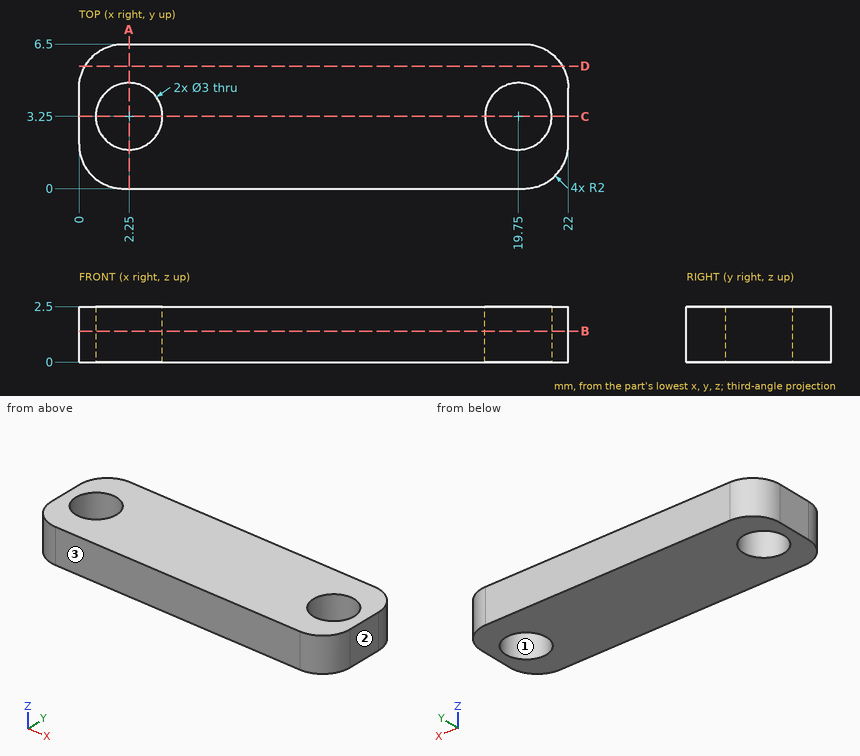
Design review of the part shown in the three views and the two pictorial views. Dimensions are in mm from the part's minimum x, y and z. Give positions to 0.01 mm unless a question says otherwise; leave off trailing zeros. Write each loop counter-clockwise with the first axis right and the second up, starting at its lowest first coordinate (ties: lowest second). Pieces come first, ordered by that corner, then holes. Notation, with made-up numbers: M 65,35.25 L 74,35.25 A26 cw 74,71.25 Z; hole C 1.5,58 d1. An arc over 180 degrees is marked long. Answer in a Markdown table with one row per item.
Item 1: For P1, Ø2.5, axis at x = 19.75, y = 3.25, coming from the -Z side, flat-tipped, find the tip position at first contact; note if it passes through.
Check sheet entries:
| item | result |
|---|---|
| P1 | through |
Item 2: Draft analysis for pull direction Y (two halves, no side actions). For the marked faces 1, 2 and 3, state which applies: +Y half, -Y half, draft (parallel to the pull), parting line (faces both ways), or undercut.
Check sheet entries:
| item | result |
|---|---|
| face 1 | undercut |
| face 2 | draft |
| face 3 | -Y half |
Item 3: Add section B-B on z = 1.4. Give the boundary of the cut face in (x, y).
Check sheet entries:
| item | result |
|---|---|
| outline | M 0,2 A2 ccw 2,0 L 20,0 A2 ccw 22,2 L 22,4.5 A2 ccw 20,6.5 L 2,6.5 A2 ccw 0,4.5 Z; hole C 2.25,3.25 d3; hole C 19.75,3.25 d3 |
Item 4: For line 1 along Y through (x, z) = (19.75, 0.75); line 2 along X through (y, z) = (2.75, 0.75); line 3 along Y through (x, z) = (18.5, 0.65), list the stretches that pass through material, from the lowest coordinate up.
Check sheet entries:
| item | result |
|---|---|
| line 1 | 0 to 1.75, 4.75 to 6.5 |
| line 2 | 0 to 0.84, 3.66 to 18.34, 21.16 to 22 |
| line 3 | 0 to 2.42, 4.08 to 6.5 |
Item 5: Add section C-C on y = 3.25. Give the boundary of the cut face in (x, z), plus the area to 3 significant figures.
Check sheet entries:
| item | result |
|---|---|
| outline | M 0,0 L 0.75,0 L 0.75,2.5 L 0,2.5 Z; M 3.75,0 L 18.25,0 L 18.25,2.5 L 3.75,2.5 Z; M 21.25,0 L 22,0 L 22,2.5 L 21.25,2.5 Z |
| area | 40.0 mm2 |
Item 6: Add section A-A on x = 2.25. Give the boundary of the cut face in (y, z).
Check sheet entries:
| item | result |
|---|---|
| outline | M 0,0 L 1.75,0 L 1.75,2.5 L 0,2.5 Z; M 4.75,0 L 6.5,0 L 6.5,2.5 L 4.75,2.5 Z |
Item 7: Add section D-D on y = 5.5. Give the boundary of the cut face in (x, z), plus the area to 3 significant figures.
Check sheet entries:
| item | result |
|---|---|
| outline | M 0.27,0 L 21.73,0 L 21.73,2.5 L 0.27,2.5 Z |
| area | 53.7 mm2 |
